Design review of the part built by this model. Coordinates are the model's own, in mm. A direction names the side the tool comes from. Coordinates: 2 decimals unless noted, no trailing zeros. Loops run counter-clockwise (first coordinate to the right, second up) from the corner with the lowest first, then second, coordinate; pieces in that order, holes last. Notation, with made-up numbers: (16, -18.5) -> (50, -18.5) arc R27 cw to (50, 10.5) -> close; hole circle Ø7 at (0.25, 7.25). An arc over 180 degrees is marked (long way). Answer as a JSON object with one key per item and string values.
Autodesk Inventor part; units mm, degrees
ref_plane "YZ Plane" through (0, 0, 0) normal (1, 0, 0) x (0, 1, 0)
ref_plane "XZ Plane" through (0, 0, 0) normal (0, 1, 0) x (-1, 0, 0)
ref_plane "XY Plane" through (0, 0, 0) normal (0, 0, 1) x (1, 0, 0)
sketch "Эскиз1" plane through (0, 0, 0) normal (1, 0, 0) x (0, 1, 0)
  circle A0 centre (0, 0) radius 5
  circle A1 centre (0, -2.7) radius 0.6
  circle A2 centre (0, 0) radius 2.7 construction
  circle A3 centre (-2.3383, 1.35) radius 0.6
  circle A4 centre (2.3383, 1.35) radius 0.6
  line L0 (0, 0) -> (5.4782, 3.1628) construction
  line L1 (0, 0) -> (-5.2011, 3.0029) construction
  line L2 (0, 0) -> (5.5612, 0) construction
  point P0 (2.3383, 1.35)
  dimension "d1" = 10
  dimension "d3" = 1.2
  dimension "d24" = 5.4
  dimension "d25" = 1.2
  dimension "d26" = 1.2
  dimension "d53" = 120
  dimension "d54" = 30
extrude "Выдавливание1" add sketch "Эскиз1" along normal blind 6 contours A0 | A3 | A4
sketch "Эскиз4" plane through (6, 0, 0) normal (1, 0, 0) x (0, 0, -1)
  circle A0 centre (2.7, 0) radius 0.6
  point P0 (-1.35, 2.3383)
  point P1 (-1.35, 2.3383)
hole "Отверстие2" at (6, 0, -2.7) direction (-1, 0, 0) diameter 1.7 depth 3
extrude "Выдавливание2" cut sketch "Эскиз1" along normal blind 6 contours A3 | A4
sketch "Эскиз2" plane through (6, 0, 0) normal (1, 0, 0) x (0, 0, -1)
  point P0 (0, 0)
  point P1 (-1.35, 2.3383)
  point P2 (-1.35, 2.3383)
hole "Отверстие4" at (6, 2.3383, 1.35) direction (-1, 0, 0) diameter 1.8 depth 3
sketch "Эскиз3" plane through (6, 0, 0) normal (1, 0, 0) x (0, 0, -1)
  point P0 (0, 0)
  point P1 (-1.35, -2.3383)
  point P2 (-1.35, -2.3383)
hole "Отверстие5" at (6, -2.3383, 1.35) direction (-1, 0, 0) diameter 1.8 depth 3
equation "\"d1\" = inside"
equation "\"d3\" = 2 * pin_small_rad"
equation "\"d17\" = pin_big_dia"
properties part number "каркас" material "Пластмасса, непрозрачная, черная"
1) For faces 1 (the cylindrical face through (4.479, 3.217, 1.545)), 2 (the cylindrical face through (1.479, -2.468, 1.936)), list the 3-axis set-ups (+Z, -Z, +X, -X, +Y, -Y) from which the entire face can be reached by the end or side of a thin tool; tool diameter is ignored.
Completed:
{"face 1": "+X", "face 2": "+X, -X"}
2) Wall thickness on probe 1 along Z at (x, y) = (1.5, 0); probe 2 along Y at (x, z) = (0.85, 1.35); probe 3 along Y at (x, z) = (1.7, -2.7): over which ranges is each line inside the solid? List them lowest first.
Completed:
{"probe 1": "-5 to -3.3, -2.1 to 5", "probe 2": "-4.81 to -2.94, -1.74 to 1.74, 2.94 to 4.81", "probe 3": "-4.21 to -0.6, 0.6 to 4.21"}
3) Add section D-D, the plane z = -2.7. Give the boundary of the cut face in (x, y).
Completed:
{"outline": "(0, -4.21) -> (6, -4.21) -> (6, -0.85) -> (3, -0.85) -> (3, -0.6) -> (0, -0.6) -> close; (0, 0.6) -> (3, 0.6) -> (3, 0.85) -> (6, 0.85) -> (6, 4.21) -> (0, 4.21) -> close"}
4) The part is to be moulded in two halves that separate along Z. For faces 3 (the flat face through (0, 0, 0)), 4 (the cylindrical face through (1.479, 1.862, 1.715)), 5 (the cylindrical face through (2.96, -1.08, 4.88)), say which applies: pulls with the +Z half, pulls with the -Z half, needs draft (parallel to the pull), parting line crosses it, or undercut.
Completed:
{"face 3": "needs draft", "face 4": "undercut", "face 5": "parting line crosses it"}
5) Clearance check with flat-ended pins moving along their axes: pin 1 Ø1.5 at (x, z) = (2, 1.5) entering from +Y; pin 2 Ø1.4 at (y, z) = (0, -2.7) entering from +X; pin 3 Ø2 at (x, z) = (1.5, -3.5) entering from -Y. State where each tip first meets the part, or that it passes through.
Completed:
{"pin 1": "y = 4.94", "pin 2": "x = 3", "pin 3": "y = -4.33"}
6) Add section C-C, the plane x = 2.8. Give the boundary of the cut face in (y, z).
Completed:
{"outline": "circle Ø10 at (0, 0); hole circle Ø1.2 at (-2.34, 1.35); hole circle Ø1.2 at (0, -2.7); hole circle Ø1.2 at (2.34, 1.35)"}
7) Add section B-B, the plane z = 1.35. Give the boundary of the cut face in (x, y), and give its area (3 significant figures).
Completed:
{"outline": "(0, -4.81) -> (6, -4.81) -> (6, -3.24) -> (3, -3.24) -> (3, -2.94) -> (0, -2.94) -> close; (0, -1.74) -> (3, -1.74) -> (3, -1.44) -> (6, -1.44) -> (6, 1.44) -> (3, 1.44) -> (3, 1.74) -> (0, 1.74) -> close; (0, 2.94) -> (3, 2.94) -> (3, 3.24) -> (6, 3.24) -> (6, 4.81) -> (0, 4.81) -> close", "area": "39.8 mm²"}
8) Add section A-A, the plane y = 0. Give the boundary of the cut face in (x, z).
Completed:
{"outline": "(0, -5) -> (6, -5) -> (6, -3.55) -> (3, -3.55) -> (3, -3.3) -> (0, -3.3) -> close; (0, -2.1) -> (3, -2.1) -> (3, -1.85) -> (6, -1.85) -> (6, 5) -> (0, 5) -> close"}
